```python
from build123d import *

# Parameters (mm, degrees)
SKETCH_2_R          = 1.385
CUT_EXTRUDE_1_DEPTH = 10
SKETCH_3_R          = 4.295
CUT_EXTRUDE_2_DEPTH = 10
SKETCH_4_W          = 5.34454344
SKETCH_4_H          = 1.293128569
EXTRUDE_1_DEPTH     = 7
SKETCH_6_R          = 1.385
CUT_EXTRUDE_3_DEPTH = 7


with BuildPart() as part:
    # 草圖1 → 旋轉1 (revolve)
    with BuildSketch(Plane.XY, mode=Mode.PRIVATE) as revolve_1_sk:
        Polygon((0, 0), (0, 19.795), (4.87, 19.795), (10.87, 10.213858447), (14.87, 10.213858447), (20.87, 19.795), (25.74, 19.795), (25.74, 10.213858447), (35.74, 10.213858447), (35.74, 0), align=None)
    revolve(revolve_1_sk.sketch.rotate(Axis((-743.15639781, 0, 0), (1, 0, 0)), 90), axis=Axis((-743.15639781, 0, 0), (1, 0, 0)))

    # 草圖2 → 除料-伸長1 (cut)
    with BuildSketch(Plane(origin=(0, 12, 0), x_dir=(1, 0, 0), z_dir=(0, 1, 0))):
        with Locations(Location((30.456485429, 0, 0), (0, 0, 270))):
            Circle(SKETCH_2_R)
    extrude(amount=-CUT_EXTRUDE_1_DEPTH, mode=Mode.SUBTRACT)

    # 草圖3 → 除料-伸長2 (cut)
    with BuildSketch(Plane(origin=(35.74, 0, 0), x_dir=(0, 0, -1), z_dir=(1, 0, 0))):
        Circle(SKETCH_3_R)
    extrude(amount=-CUT_EXTRUDE_2_DEPTH, mode=Mode.SUBTRACT)

    # 草圖4 → 填料-伸長1 (add)
    with BuildSketch(Plane(origin=(25.74, 0, 0), x_dir=(0, 0, -1), z_dir=(1, 0, 0))):
        with Locations((-0.084600543, 4.07453495)):
            Rectangle(SKETCH_4_W, SKETCH_4_H)
    extrude(amount=EXTRUDE_1_DEPTH)

    # 草圖6 → 除料-伸長3 (cut)
    with BuildSketch(Plane(origin=(0, 4.721099234, 0), x_dir=(1, 0, 0), z_dir=(0, 1, 0))):
        with Locations(Location((30.456485429, 0, 0), (0, 0, 270))):
            Circle(SKETCH_6_R)
    extrude(amount=-CUT_EXTRUDE_3_DEPTH, mode=Mode.SUBTRACT)


solid = part.part
```
Check sheet for the modelled part. Datum: model origin and axes. Units: mm. A direction names the side the tool comes from. Give positions to 0.01 mm unless a question says otherwise; leave off trailing zeros. Write each loop counter-clockwise with the first axis right and the second up, starting at its lowest first coordinate (ties: lowest second). Pieces come first, ordered by that corner, then holes. Notation, with made-up numbers: (56.5, 78.25) - (78.5, 78.25) arc R28 cw to (78.5, 98.25) - close; hole circle Ø3 at (41.25, 11.5). An arc over 180 degrees is marked (long way). Answer as a JSON object with one key per item and string values. Group by question number.
1) Thickness scan on probe 1 along X at (y, z) = (6, 0); probe 2 along X at (y, z) = (11, 9.5); probe 3 along Y at (x, z) = (31, 0) (3 decimals). Record the ranges inside material, lowest first. Write a range as from..to.
2) Release check for a two-part mould opening along Y. For faces 1 (the face through (25.74, 9, 9)), 2 (the face through (30.8, -4.2, 0.9)), 3 (the face through (30.81, -3.07, 9.74)) record: pulls with the +Y half, pulls with the -Y half, needs draft (parallel to the pull), parting line crosses it, or undercut.
3) Sectioned sample at C-C (x = 24.5). Record the cut outline in (y, z) (3 decimals), then the cut area to 3 significant figures.
4) Sectioned sample at D-D (x = 7.5). Record the cut outline in (y, z), then the cut area to 3 significant figures.
5) Access from +Z, -Z, +X, -X, +Y, -Y to the whole of each face (thin tool, end or side, straight path). Record for faces 4 (the face through (10.579, -10.588, -1.39)), 5 (the face through (28, 3.428, 0)), 6 (the face through (31.83, 6.87, -0.18)).
6) Sectioned sample at B-B (y = 0). Record the cut outline in (x, z) (3 decimals).
7) Sectioned sample at A-A (z = 0). Record the cut outline in (x, y) (3 decimals).
8) Depth check by flat-ended pin: P1, Ø3, axis at x = 30.46, z = 0, coming from the +Y side; P2, Ø5.5, axis at x = 28, z = 0, coming from the -Y side (3 decimals); P3, Ø8, axis at x = 26, y = 12, coming from the -Z side. Enter the tip coordinate at first touch or a pass-through.
Geometry results:
{
 "1": {"probe 1": "x = 0..29.07, 31.84..35.74", "probe 2": "x = 0..8.16, 17.58..25.74", "probe 3": "y = -10.214..-4.295"},
 "2": {"face 1": "needs draft", "face 2": "undercut", "face 3": "parting line crosses it"},
 "3": {"outline": "circle Ø39.59 at (0, 0)", "area": "1,230 mm^2"},
 "4": {"outline": "circle Ø31.19 at (0, 0)", "area": "764 mm^2"},
 "5": {"face 4": "none", "face 5": "+X", "face 6": "+Y"},
 "6": {"outline": "(0, -19.795) - (4.87, -19.795) - (10.87, -10.214) - (14.87, -10.214) - (20.87, -19.795) - (25.74, -19.795) - (25.74, -10.214) - (35.74, -10.214) - (35.74, -4.295) - (25.74, -4.295) - (25.74, 4.295) - (35.74, 4.295) - (35.74, 10.214) - (25.74, 10.214) - (25.74, 19.795) - (20.87, 19.795) - (14.87, 10.214) - (10.87, 10.214) - (4.87, 19.795) - (0, 19.795) - close"},
 "7": {"outline": "(0, -19.795) - (4.87, -19.795) - (10.87, -10.214) - (14.87, -10.214) - (20.87, -19.795) - (25.74, -19.795) - (25.74, -10.214) - (35.74, -10.214) - (35.74, -4.295) - (25.74, -4.295) - (25.74, 3.428) - (29.071, 3.428) - (29.071, 10.214) - (25.74, 10.214) - (25.74, 19.795) - (20.87, 19.795) - (14.87, 10.214) - (10.87, 10.214) - (4.87, 19.795) - (0, 19.795) - close; (31.841, 3.428) - (32.74, 3.428) - (32.74, 4.295) - (35.74, 4.295) - (35.74, 10.214) - (31.841, 10.214) - close"},
 "8": {"P1": "stops at y = 10.21", "P2": "stops at y = -19.795", "P3": "stops at z = -18.1"}
}
